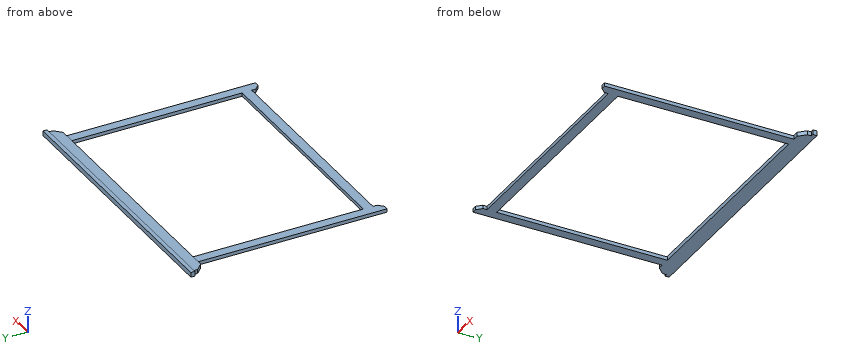
```python
from build123d import *

# Parameters (mm, degrees)
F1_DEPTH = 30
F0_W     = 20
F0_H     = 30
F0_W_2   = 1960
F2_DEPTH = 35
F0_W_3   = 1640
F0_H_2   = 70
F3_DEPTH = 25


with BuildPart() as f1:
    # F0 (on Top) → F1 (new body)
    with BuildSketch(Plane.XY):
        Polygon((-1947.5297451019, -160.4416549206), (-1877.5297451019, -160.4416549206), (-237.5297451019, -160.4416549206), (-167.5297451019, -160.4416549206), (-127.5297451019, -160.4416549206), (-77.5297451019, -110.4416549206), (-77.5297451019, -80.4416549206), (-2037.5297451019, -80.4416549206), (-2037.5297451019, -110.4416549206), (-1987.5297451019, -160.4416549206), align=None)
    extrude(amount=F1_DEPTH)

    # F0 (on Top) → F2 (join)
    with BuildSketch(Plane.XY):
        with Locations((-2047.5297451019, -65.4416549206)):
            Rectangle(F0_W, F0_H)
        with Locations((-1057.5297451019, -65.4416549206)):
            Rectangle(F0_W_2, F0_H)
        with Locations((-67.5297451019, -65.4416549206)):
            Rectangle(F0_W, F0_H)
    extrude(amount=F2_DEPTH)

    # F0 (on Top) → F3 (join)
    with BuildSketch(Plane.XY):
        Polygon((-1877.5297451019, -1410.4416549206), (-1877.5297451019, -160.4416549206), (-1947.5297451019, -160.4416549206), (-1947.5297451019, -1545.4416549206), (-1912.5297451019, -1545.4416549206), (-1877.5297451019, -1510.4416549206), (-1877.5297451019, -1480.4416549206), align=None)
        with Locations((-1057.5297451019, -1445.4416549206)):
            Rectangle(F0_W_3, F0_H_2)
        Polygon((-167.5297451019, -160.4416549206), (-237.5297451019, -160.4416549206), (-237.5297451019, -1410.4416549206), (-237.5297451019, -1480.4416549206), (-237.5297451019, -1510.4416549206), (-202.5297451019, -1545.4416549206), (-167.5297451019, -1545.4416549206), align=None)
    extrude(amount=F3_DEPTH)


solid = f1.part
```
For this review, take the finished solid that the model builds, in its own axes (mm). Round coordinates to 2 decimals unless told otherwise and drop trailing zeros. Write each loop counter-clockwise with the first axis right and the second up, starting at its lowest first coordinate (ties: lowest second). Pieces come first, ordered by that corner, then holes. Notation, with made-up numbers: (45, 53) -> (91, 53) arc R14 cw to (91, 64) -> close; hole circle Ø2 at (-28, -15.5). An arc over 180 degrees is marked (long way). One line per question, with ' | ' between items. Start each with the question number.
1) Add section C-C (y = -351.5). Write out the cut boundary in (x, z), and give its area (3 significant figures).
2) Add section B-B (x = -1007.5). Write out the cut boundary in (y, z), and give its area (3 significant figures).
3) For pin 1 Ø7.5 at (y, z) = (-796, 11) entering from -X; pin 2 Ø6 at (y, z) = (-325.5, 26.5) entering from +X; pin 3 Ø9 at (y, z) = (-88.5, 11) entering from +X, all flat-tipped, find the tip position at first contact; note any pin that passes through.
4) Wall thickness on line 1 along X through (y, z) = (-649, 15); line 2 along Y through (x, z) = (-1528, 2); line 3 along Y through (x, z) = (-271, 29): over which ranges is each line inside the solid? List them lowest first.
5) Add section A-A (z = 10). Write out the cut boundary in (x, y), and give its area (3 significant figures).
Reported:
1) outline: (-1947.53, 0) -> (-1877.53, 0) -> (-1877.53, 25) -> (-1947.53, 25) -> close; (-237.53, 0) -> (-167.53, 0) -> (-167.53, 25) -> (-237.53, 25) -> close | area: 3,500 mm²
2) outline: (-1480.44, 0) -> (-1410.44, 0) -> (-1410.44, 25) -> (-1480.44, 25) -> close; (-160.44, 0) -> (-50.44, 0) -> (-50.44, 35) -> (-80.44, 35) -> (-80.44, 30) -> (-160.44, 30) -> close | area: 5,200 mm²
3) pin 1: stops at x = -1947.53 | pin 2: stops at x = -167.53 | pin 3: stops at x = -77.53
4) line 1: x = -1947.53 to -1877.53, -237.53 to -167.53 | line 2: y = -1480.44 to -1410.44, -160.44 to -50.44 | line 3: y = -160.44 to -50.44
5) outline: (-2057.53, -80.44) -> (-2037.53, -80.44) -> (-2037.53, -110.44) -> (-1987.53, -160.44) -> (-1947.53, -160.44) -> (-1947.53, -1545.44) -> (-1912.53, -1545.44) -> (-1877.53, -1510.44) -> (-1877.53, -1480.44) -> (-237.53, -1480.44) -> (-237.53, -1510.44) -> (-202.53, -1545.44) -> (-167.53, -1545.44) -> (-167.53, -160.44) -> (-127.53, -160.44) -> (-77.53, -110.44) -> (-77.53, -80.44) -> (-57.53, -80.44) -> (-57.53, -50.44) -> (-2057.53, -50.44) -> close; hole (-1877.53, -1410.44) -> (-237.53, -1410.44) -> (-237.53, -160.44) -> (-1877.53, -160.44) -> close | area: 522,000 mm²
